Verification items for this drawing (mm, ordinates from the low corner). A direction names the side the tool comes from. Round coordinates to 2 decimals unless told otherwise and drop trailing zeros. Order: outer loops, then holes, each group sorted by start corner. A loop starts at its lowest first (then second) coordinate and runs counter-clockwise, first axis right, second up.
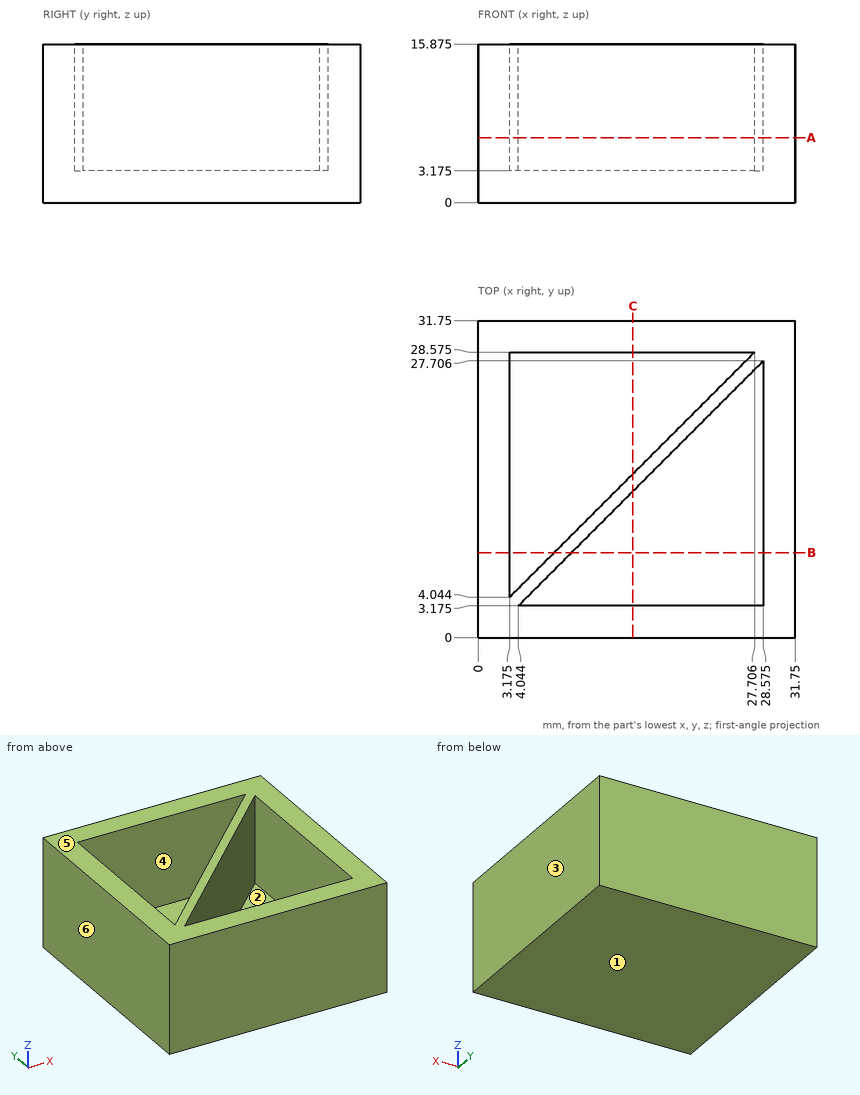
Item 1: Access from +Z, -Z, +X, -X, +Y, -Y to the whole of each face (thin tool, end or side, straight path). Record for the marked faces 1 and 2.
Answer:
face 1: -Z, +X, -X, +Y, -Y
face 2: +Z
Item 2: Scan line: line 1 along Z through (x, y) = (10.5, 28) (3 decimals). Record every from-to range of solid material in increasing order.
Answer:
line 1: z = 0 to 3.175
Item 3: Sectioned sample at B-B (y = 8.5). Record the cut outline in (x, z) (3 decimals).
Answer:
outline: (0, 0) - (31.75, 0) - (31.75, 15.875) - (28.575, 15.875) - (28.575, 3.175) - (9.369, 3.175) - (9.369, 15.875) - (7.631, 15.875) - (7.631, 3.175) - (3.175, 3.175) - (3.175, 15.875) - (0, 15.875) - close
Item 4: Release check for a two-part mould opening along X. For the marked faces 3, 4, 5 and 6 record: released by +X, released by -X, zero draft, split by the parting line, or undercut.
Answer:
face 3: released by +X
face 4: undercut
face 5: zero draft
face 6: released by -X
Item 5: Sectioned sample at C-C (x = 15.5). Record the cut outline in (y, z) (3 decimals), and give its area (3 significant figures).
Answer:
outline: (0, 0) - (31.75, 0) - (31.75, 15.875) - (28.575, 15.875) - (28.575, 3.175) - (16.369, 3.175) - (16.369, 15.875) - (14.631, 15.875) - (14.631, 3.175) - (3.175, 3.175) - (3.175, 15.875) - (0, 15.875) - close
area: 204 mm2
Item 6: Sectioned sample at A-A (z = 6.5). Record the cut outline in (x, y) (3 decimals), and give its area (3 significant figures).
Answer:
outline: (0, 0) - (31.75, 0) - (31.75, 31.75) - (0, 31.75) - close; hole (3.175, 4.044) - (27.706, 28.575) - (3.175, 28.575) - close; hole (4.044, 3.175) - (28.575, 3.175) - (28.575, 27.706) - close
area: 406 mm2
